```python
from build123d import *

# Parameters (mm, degrees)
F0_W           = 11.4
F0_H           = 57.9
F0_W_2         = 27
F0_H_2         = 18.9
F0_W_3         = 16.7
F0_H_3         = 17.6
F1_DEPTH       = 3.175
F5_D           = 4.4
F5_DEPTH       = 12
F5_TIP         = 1.3218933619
F6_D           = 4.4
F6_DEPTH       = 12
F6_TIP         = 1.3218933619
F6_ON_F4_D     = 4.4
F6_ON_F4_DEPTH = 12
F6_ON_F4_TIP   = 1.3218933619
F8_D           = 3.3


# Not quite as in the source:
# - a feature names something its author has since deleted; it is built from what else it names


with BuildPart() as f1:
    # F0 (on Front) → F1 (new body, symmetric)
    with BuildSketch(Plane.XZ):
        Polygon((163, -200), (203, -200), (203, 200), (-203, 200), (-203, -200), (-183, -200), (-183, -95), (37, -95), (37, -200), (68, -200), (68, -91.22133255), (163, -91.22133255), align=None)
        with Locations((-162.4, 51.05)):
            Rectangle(F0_W, F0_H, mode=Mode.SUBTRACT)
        with Locations((-132.4, 51.05)):
            Rectangle(F0_W, F0_H, mode=Mode.SUBTRACT)
        with Locations((-102.4, 51.05)):
            Rectangle(F0_W, F0_H, mode=Mode.SUBTRACT)
        with Locations((-72.4, 51.05)):
            Rectangle(F0_W, F0_H, mode=Mode.SUBTRACT)
        with Locations((-42.4, 51.05)):
            Rectangle(F0_W, F0_H, mode=Mode.SUBTRACT)
        with Locations((-12.4, 51.05)):
            Rectangle(F0_W, F0_H, mode=Mode.SUBTRACT)
        with Locations((17.6, 51.05)):
            Rectangle(F0_W, F0_H, mode=Mode.SUBTRACT)
        with Locations((47.6, 51.05)):
            Rectangle(F0_W, F0_H, mode=Mode.SUBTRACT)
        with Locations((77.6, 51.05)):
            Rectangle(F0_W, F0_H, mode=Mode.SUBTRACT)
        with Locations((119.8, 31.55)):
            Rectangle(F0_W_2, F0_H_2, mode=Mode.SUBTRACT)
        with Locations((164.65, 30.9)):
            Rectangle(F0_W_3, F0_H_3, mode=Mode.SUBTRACT)
        with Locations((119.8, 70.55)):
            Rectangle(F0_W_2, F0_H_2, mode=Mode.SUBTRACT)
        with Locations((164.65, 71.2)):
            Rectangle(F0_W_3, F0_H_3, mode=Mode.SUBTRACT)
    extrude(amount=F1_DEPTH, both=True)

    # F5
    with Locations(Plane.XY.offset(200)):
        with Locations((-183, 0), (0, 0), (183, 0)):
            Hole(F5_D / 2, depth=F5_DEPTH)
            with Locations((0, 0, -(F5_DEPTH + F5_TIP / 2))):  # 118° drill point
                Cone(0, F5_D / 2, F5_TIP, mode=Mode.SUBTRACT)

    # F6
    with Locations(Plane(origin=(-203, 0, 0), x_dir=(0, -1, 0), z_dir=(-1, 0, 0))):
        with Locations((0, -180), (0, -20), (0, 20), (0, 180)):
            Hole(F6_D / 2, depth=F6_DEPTH)
            with Locations((0, 0, -(F6_DEPTH + F6_TIP / 2))):  # 118° drill point
                Cone(0, F6_D / 2, F6_TIP, mode=Mode.SUBTRACT)

    # F6 on F4
    with Locations(Plane.YZ.offset(203)):
        with Locations((0, -180), (0, -20), (0, 20), (0, 180)):
            Hole(F6_ON_F4_D / 2, depth=F6_ON_F4_DEPTH)
            with Locations((0, 0, -(F6_ON_F4_DEPTH + F6_ON_F4_TIP / 2))):  # 118° drill point
                Cone(0, F6_ON_F4_D / 2, F6_ON_F4_TIP, mode=Mode.SUBTRACT)

    # F8 (through all)
    with Locations(Plane.XZ.offset(3.175)):
        with Locations((63, -87.5), (168, -87.5), (168, -192.5), (63, -192.5), (77.6, 82.8), (47.6, 82.8), (77.6, 19.3), (47.6, 19.3), (17.6, 19.3), (17.6, 82.8), (-12.4, 82.8), (-12.4, 19.3), (-42.4, 19.3), (-42.4, 82.8), (-72.4, 82.8), (-72.4, 19.3), (-102.4, 19.3), (-102.4, 82.8), (-132.4, 82.8), (-132.4, 19.3), (-162.4, 19.3), (-162.4, 82.8), (139.55, 70.55), (100.05, 70.55), (100.05, 31.55), (139.55, 31.55)):
            Hole(F8_D / 2)


solid = f1.part
```
Can you work these out from the model? Positions are in its coordinate system, mm. Round coordinates to 2 decimals unless told otherwise and drop trailing zeros. Loops run counter-clockwise (first coordinate to the right, second up) from the corner with the lowest first, then second, coordinate; pieces in that order, holes last. Notation, with made-up numbers: (44.5, 6) -> (58.5, 6) arc R23 cw to (58.5, 40) -> close; hole circle Ø7 at (-8, -39.75). An arc over 180 degrees is marked (long way). Answer in a Markdown table with one row per item.
Item 1: Suppose I cut it at A-A, the plane z = -158. List the corners of the cut face in (x, y) for me (3 decimals), plus the area to 3 significant figures.
Answer block:
| item | result |
|---|---|
| outline | (-203, -3.175) -> (-183, -3.175) -> (-183, 3.175) -> (-203, 3.175) -> close; (37, -3.175) -> (68, -3.175) -> (68, 3.175) -> (37, 3.175) -> close; (163, -3.175) -> (203, -3.175) -> (203, 3.175) -> (163, 3.175) -> close |
| area | 578 mm² |
Item 2: Suppose I cut it at B-B, the plane z = 54. Give the number of separate pieces and of enclosed holes in the cut face, plus the area to 3 significant figures.
Answer block:
| item | result |
|---|---|
| separate pieces | 10 |
| enclosed holes | 0 |
| area | 1,930 mm² |
Item 3: If I drill on probe 1 along X at (y, z) = (-2.75, -156); probe 2 along X at (y, z) = (0, -192.5); probe 3 along Z at (x, y) = (77.6, -0.25), over which ranges is the centre line in solid material (lowest first)?
Answer block:
| item | result |
|---|---|
| probe 1 | -203 to -183, 37 to 68, 163 to 203 |
| probe 2 | -203 to -183, 37 to 61.35, 64.65 to 68, 163 to 166.35, 169.65 to 203 |
| probe 3 | -91.22 to 17.65, 20.95 to 22.1, 80 to 81.15, 84.45 to 200 |
Item 4: Will these pins go through, and if not, where does the flat tip stop? P1, Ø3.5, axis at y = 0, z = -20, coming from the +X side; P2, Ø1, axis at x = -9, y = 0, coming from the -Z side.
Answer block:
| item | result |
|---|---|
| P1 | x = 190.73 |
| P2 | z = -95 |
